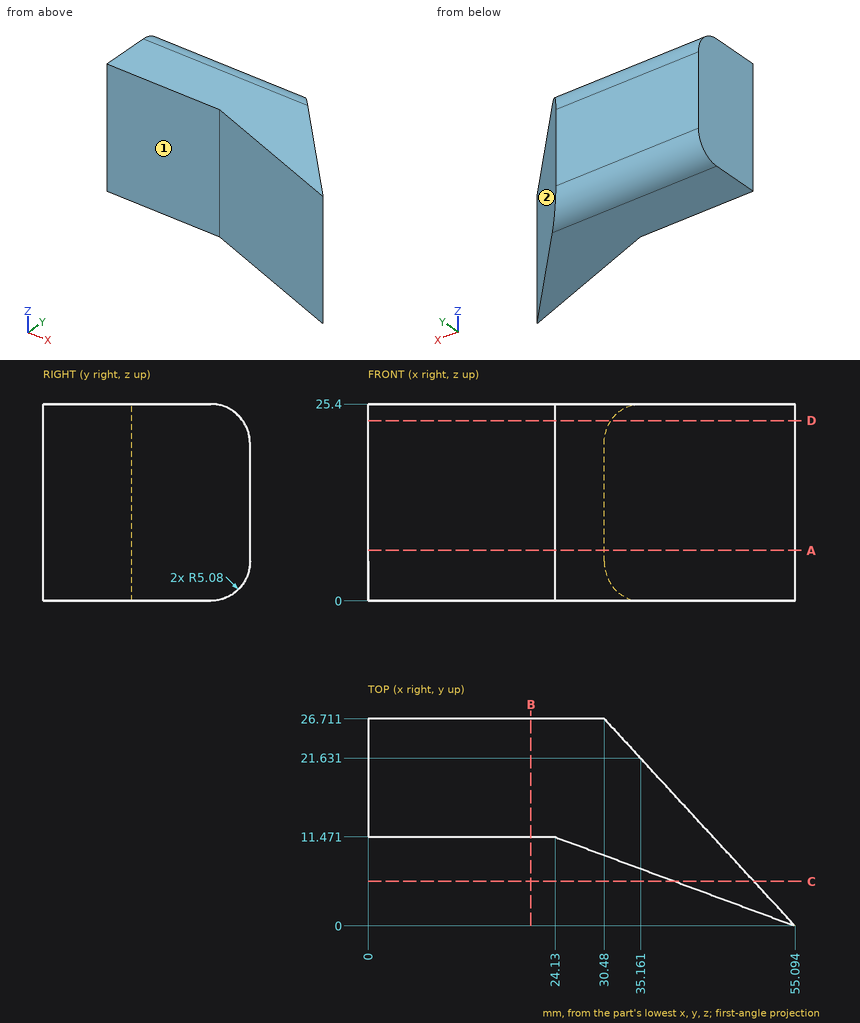
Could you check a few things on this drawing? It's one solid part, dimensions in mm from its lowest x, y, z. A direction names the side the tool comes from. Round coordinates to 2 decimals unless told otherwise and drop trailing zeros. Loops run counter-clockwise (first coordinate to the right, second up) from the corner with the lowest first, then second, coordinate; pieces in that order, holes last. Notation, with made-up numbers: (84.5, 73.5) -> (130.5, 73.5) arc R32 ccw to (130.5, 109.5) -> close; hole circle Ø3 at (34, 63.5). An arc over 180 degrees is marked (long way). One line per item, written item: value. Start each with the question number.
1. If we section it at A-A, the plane z = 6.5: Write out the boundary of the cut face in (x, y).
2. If we section it at D-D, the plane z = 23.25: Write out the boundary of the cut face in (x, y).
3. For pin 1 (8 mm diameter, centred on x = 9, z = 9, fed in from -Y); pin 2 (5 mm diameter, centred on x = 20.5, y = 10.5, fed in from +Z); pin 3 (1 mm diameter, centred on x = 45.5, z = 6.5, fed in from +Y) (1 decimal); pin 4 (10 mm diameter, centred on x = 27, z = 10, fed in from -Y) (1 decimal), each with a flat end and sliding along its axis, tell me the tip position at first contact or that it passes through.
4. If we section it at C-C, the plane y = 5.75: Write out the boundary of the cut face in (x, z) (1 decimal).
5. If we section it at B-B, the plane x = 21: Write out the boundary of the cut face in (y, z), then the cut area to 3 significant figures.
6. If I drill on probe 1 along Y at (x, z) = (14, 14.75); probe 2 along Y at (x, z) = (24.5, 18); probe 3 along X at (y, z) = (19.25, 22.75) (1 decimal), over which ranges is the centre line in solid material (lowest first)?
7. For the marked faces 1 and 2, which set-ups out of +Z, -Z, +X, -X, +Y, -Y let a thin tool reach every point of the face, with its end or its side?
Calculated:
1. outline: (0, 11.47) -> (24.13, 11.47) -> (55.09, 0) -> (30.48, 26.71) -> (0, 26.71) -> close
2. outline: (0, 11.47) -> (24.13, 11.47) -> (55.09, 0) -> (31.34, 25.78) -> (0, 25.78) -> close
3. pin 1: stops at y = 11.47
3. pin 2: stops at z = 25.4
3. pin 3: stops at y = 11
3. pin 4: stops at y = 8.6
4. outline: (39.6, 0) -> (49.8, 0) -> (49.8, 25.4) -> (39.6, 25.4) -> close
5. outline: (11.47, 0) -> (21.63, 0) arc R5.08 ccw to (26.71, 5.08) -> (26.71, 20.32) arc R5.08 ccw to (21.63, 25.4) -> (11.47, 25.4) -> close
5. area: 376 mm²
6. probe 1: y = 11.47 to 26.71
6. probe 2: y = 11.33 to 26.71
6. probe 3: x = 0 to 37.4
7. face 1: +Z, -Z, -X, -Y
7. face 2: +Z, -Z, +X, +Y
